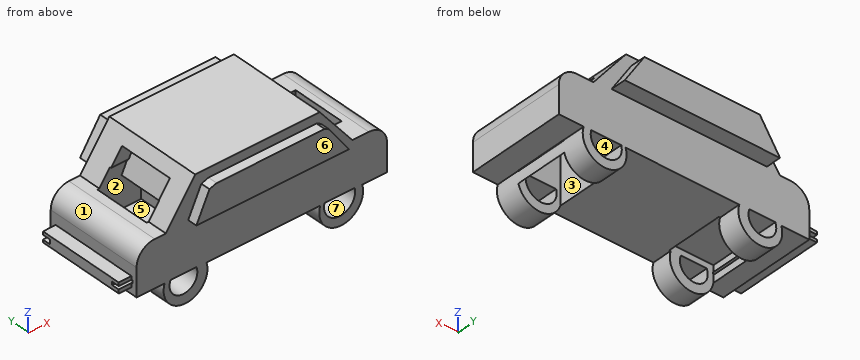
from build123d import *

# Parameters (mm, degrees)
F1_DEPTH  = 34.798
F2_W      = 14.652997
F2_H      = 18.606977
F2_W_2    = 15.350757
F2_H_2    = 20.002499
F3_DEPTH  = 33.02
F4_W      = 19.40675
F4_H      = 9.867839
F5_DEPTH  = 230.124
F6_W      = 18.839565
F6_H      = 7.907965
F7_DEPTH  = 125.476
F9_DEPTH  = 83.566
F11_DEPTH = 38.1
F13_DEPTH = 5.334
F14_W     = 30.701512
F14_H     = 3.605101
F15_DEPTH = 51.562
F16_W     = 3.986457
F16_H     = 1.545359
F17_DEPTH = 90.932
F18_W     = 3.111688
F18_H     = 1.106378
F19_DEPTH = 112.1664


with BuildPart() as f1:
    # F0 (on Front) → F1 (new body)
    with BuildSketch(Plane.XZ):
        Polygon((-26.631236, 9.187195), (-36.865074, -5.233212), (28.259346, -5.233212), (16.862571, 9.187195), align=None)
        with BuildLine():
            Line((-36.865074, -5.233212), (-40.748909, -5.233212))
            ThreePointArc((-40.748909, -5.233212), (-45.239037, -7.093084), (-47.098909, -11.583212))
            Line((-47.098909, -11.583212), (-47.098909, -21.28173))
            Line((-47.098909, -21.28173), (-37.335627, -21.28173))
            ThreePointArc((-37.335627, -21.28173), (-30.008619, -31.171456), (-22.681611, -21.28173))
            Line((-22.681611, -21.28173), (17.029377, -21.28173))
            ThreePointArc((17.029377, -21.28173), (24.356385, -31.171456), (31.683393, -21.28173))
            Line((31.683393, -21.28173), (40.353883, -21.28173))
            Line((40.353883, -21.28173), (40.353883, -11.583212))
            ThreePointArc((40.353883, -11.583212), (38.494011, -7.093084), (34.003883, -5.233212))
            Line((34.003883, -5.233212), (28.259346, -5.233212))
            Line((28.259346, -5.233212), (-36.865074, -5.233212))
        make_face()
    extrude(amount=F1_DEPTH)

    # F2 (on Top) → F3 (cut)
    with BuildSketch(Plane.XY):
        with Locations((24.421658, -17.09516)):
            Rectangle(F2_W, F2_H)
        with Locations((-29.887457, -17.792921)):
            Rectangle(F2_W_2, F2_H_2)
    extrude(amount=-F3_DEPTH, mode=Mode.SUBTRACT)

    # F4 (on Right) → F5 (cut)
    with BuildSketch(Plane.YZ):
        with Locations((-17.967003, 0.447439)):
            Rectangle(F4_W, F4_H)
    extrude(amount=-F5_DEPTH, mode=Mode.SUBTRACT)

    # F6 (on Right) → F7 (cut)
    with BuildSketch(Plane.YZ):
        with Locations((-16.978866, 0.116294)):
            Rectangle(F6_W, F6_H)
    extrude(amount=F7_DEPTH, mode=Mode.SUBTRACT)

    # F8 (on Front) → F9 (cut)
    with BuildSketch(Plane.XZ):
        with BuildLine():
            Line((-26.203193, -21.146845), (-35.248715, -21.146845))
            ThreePointArc((-35.248715, -21.146845), (-30.725954, -27.770875), (-26.203193, -21.146845))
        make_face()
        with BuildLine():
            ThreePointArc((18.531013, -21.146845), (23.793861, -27.908914), (29.056709, -21.146845))
            Line((29.056709, -21.146845), (18.531013, -21.146845))
        make_face()
    extrude(amount=F9_DEPTH, mode=Mode.SUBTRACT)

    # F10 (on Front) → F11 (join)
    with BuildSketch(Plane.XZ):
        Polygon((-24.474356, 5.173787), (-29.079348, -4.529587), (24.206989, -4.529587), (17.299499, 5.173787), (15.737092, 5.996108), (-22.007396, 5.996108), align=None)
    extrude(amount=F11_DEPTH)

    # F12 (on Front) → F13 (join)
    with BuildSketch(Plane.XZ):
        Polygon((21.933926, -4.508358), (15.019068, 6.278823), (-25.225412, 6.278823), (-32.278571, -4.508358), align=None)
    extrude(amount=-F13_DEPTH)

    # F14 (on Right) → F15 (join)
    with BuildSketch(Plane.YZ):
        with Locations((-17.393864, -17.231901)):
            Rectangle(F14_W, F14_H)
    extrude(amount=-F15_DEPTH)

    # F16 (on Right) → F17 (cut)
    with BuildSketch(Plane.YZ):
        with Locations((-2.872, -17.325192)):
            Rectangle(F16_W, F16_H)
    extrude(amount=-F17_DEPTH, mode=Mode.SUBTRACT)

    # F18 (on Right) → F19 (cut)
    with BuildSketch(Plane.YZ):
        with Locations((-31.648566, -17.165717)):
            Rectangle(F18_W, F18_H)
    extrude(amount=-F19_DEPTH, mode=Mode.SUBTRACT)


solid = f1.part
CAD build for the part. Positions are in the model's coordinates, mm. Face numbers are marked on the shaded views. A direction names the side the tool comes from. Give positions to 0.01 mm unless a question says otherwise; leave off trailing zeros. Write each loop counter-clockwise with the first axis right and the second up, starting at its lowest first coordinate (ties: lowest second). Pieces come first, ordered by that corner, then holes. Notation, with made-up numbers: M 39.25,-9.5 L 80.25,-9.5 A11 cw 80.25,5.5 Z; hole C 41.25,32 d7. An arc over 180 degrees is marked long. Put each result on its own line as item: value. Start each with the question number.
(1) Band-saw the part on C-C, the plane y = -15. Give the number of separate pieces and of enclosed holes in the cut face, and give its area (3 significant figures).
(2) Flat gauge pins, fed straight in: pin 1 Ø1 at (x, y) = (-13.5, -37) entering from -Z; pin 2 Ø10 at (x, z) = (29, 4) entering from -Y; pin 3 Ø0.8 at (y, z) = (-2.5, -17) entering from -X; pin 4 Ø0.9 at (x, z) = (-17, -17.5) entering from +Y. Where does each tip first touch, or does it go through?
(3) Which spindle directions (+Z, -Z, +X, -X, +Y, -Y) get a long thin tool onto all of the face, cutting with end or side? Do the marked faces 1, 2, 3 and 4. Say none if no direction does.
(4) Band-saw the part on D-D, the plane y = 2. Write the cut outline in (x, z), and give its area (3 significant figures).
(5) Mould opens along Y. For the marked faces 5, 6 and 7 say: +Y half, -Y half, draft (parallel to the pull), parting line (faces both ways), or undercut.
(6) Band-saw the part on B-B, the plane x = 7. Write the cut outline in (y, z).
(7) Band-saw the part on A-A, the plane x = -11.5. Write the cut outline in (y, z), and give its area (3 significant figures).
(8) Probe L1, parallel to X at y = -12, z = -14.5; L2, parallel to Y at x = 26.5, z = -5.5; L3, parallel to Y at x = -46, z = -17. List the from-to ranges inside material, lowest first.
Response values:
1. separate pieces: 4
1. enclosed holes: 0
1. area: 1,660 mm2
2. pin 1: stops at z = -4.53
2. pin 2: passes through
2. pin 3: stops at x = 0
2. pin 4: stops at y = 0
3. face 1: +Z, -X, +Y, -Y
3. face 2: none
3. face 3: -Z
3. face 4: +Y, -Y
4. outline: M -32.28,-4.51 L 21.93,-4.51 L 15.02,6.28 L -25.23,6.28 Z
4. area: 509 mm2
5. face 5: undercut
5. face 6: -Y half
5. face 7: draft
6. outline: M -38.1,-4.53 L -34.8,-4.53 L -34.8,-21.28 L 0,-21.28 L 0,-4.51 L 5.33,-4.51 L 5.33,6.28 L 0,6.28 L 0,9.19 L -34.8,9.19 L -34.8,6 L -38.1,6 Z
7. outline: M -38.1,-4.53 L -34.8,-4.53 L -34.8,-21.28 L 0,-21.28 L 0,-4.51 L 5.33,-4.51 L 5.33,6.28 L 0,6.28 L 0,9.19 L -34.8,9.19 L -34.8,6 L -38.1,6 Z; hole M -33.2,-17.72 L -30.09,-17.72 L -30.09,-16.61 L -33.2,-16.61 Z; hole M -4.87,-18.1 L -0.88,-18.1 L -0.88,-16.55 L -4.87,-16.55 Z
7. area: 1,140 mm2
8. L1: x = -47.1 to -37.56, -22.21 to 17.1, 31.75 to 40.35
8. L2: y = -34.8 to -26.4, -7.79 to 0
8. L3: y = -34.8 to -33.2, -30.09 to -4.87, -0.88 to 0
